Build history of the part. All positions in model axes, mm. A direction names the side the tool comes from. Coordinates: 2 decimals unless noted, no trailing zeros. Loops run counter-clockwise (first coordinate to the right, second up) from the corner with the lowest first, then second, coordinate; pieces in that order, holes last.
(1) Two-plate mould, pull along Y, no slides. Class faces 4 (the face through (45.66, 34.61, 4.93)), 5 (the face through (-0.243, -30.316, 4.93)), 6 (the face through (46.185, -35.23, 4.93)), 7 (the face through (0, 0, 100)): pulls with the +Y half, pulls with the -Y half, needs draft (parallel to the pull), parting line crosses it, or undercut.
(2) Slice it at A-A (x = 0). Give the cut face in (y, z).
(3) Tool access for faces 1 (the face through (-30.57, -55.48, 4.93)), 2 (the face through (-45.66, -34.61, 4.93)), 3 (the face through (6.691, -12.864, 54.37)): list every direction of +Z, -Z, +X, -X, +Y, -Y with a clear straight run to the whole face (end or side of a thin tool).
(4) Slice it at D-D (z = 80). Give the cut face in (x, y).
(5) Slice it at C-C (y = -32.5). Give the cut face in (x, z), and give its area (3 significant figures).
(6) Slice it at B-B (y = 0). Give the cut face in (x, z).
(7) Wall check: L1, parallel to Z at x = 0, y = -1.5; L2, parallel to X at y = -0.5, z = 90.5; L3, parallel to Z at x = -47.5, y = 67. Give the ranges that are in metal, low to high.
(8) Flat gauge pins, fed straight in: P1, Ø6, axis at x = 6.5, z = 75.5, coming from the -Y side; P2, Ø8, axis at x = 25.5, y = 60, coming from the +Z side; P3, Ø16, axis at x = 0, z = 80, coming from the -Y side; P4, Ø6, axis at x = -48, y = 45, coming from the +Z side. Where does each tip first touch, or does it go through?
from build123d import *

# Parameters (mm, degrees)
F1_DEPTH = 10
F3_R     = 14.5
F4_DEPTH = 90
F2_R     = 5
F5_DEPTH = 25


# Not quite as in the source:
# - a feature names something its author has since deleted; it is built from what else it names


with BuildPart() as f1:
    # F0 (on Top) → F1 (new body)
    with BuildSketch(Plane.XY):
        with BuildLine():
            Line((-45.4576714329, 73.0742780183), (-55, 65))
            Line((-55, 65), (-46.9257219817, 55.4576714329))
            ThreePointArc((-46.9257219817, 55.4576714329), (-43.6602805319, 59.7406500035), (-42.5, 65))
            ThreePointArc((-42.5, 65), (-43.2626854202, 69.2994704855), (-45.4576714329, 73.0742780183))
        make_face()
        with BuildLine():
            Line((-46.9257219817, 55.4576714329), (-55, 65))
            Line((-55, 65), (-64.5423285671, 56.9257219817))
            ThreePointArc((-64.5423285671, 56.9257219817), (-56.0380684982, 52.5431780219), (-46.9257219817, 55.4576714329))
        make_face()
        with BuildLine():
            Line((-64.5423285671, 56.9257219817), (-55, 65))
            Line((-55, 65), (-45.4576714329, 73.0742780183))
            ThreePointArc((-45.4576714329, 73.0742780183), (-63.0742780183, 74.5423285671), (-64.5423285671, 56.9257219817))
        make_face()
        with BuildLine():
            ThreePointArc((-42.5, 65), (-43.6602805319, 59.7406500035), (-46.9257219817, 55.4576714329))
            Line((-46.9257219817, 55.4576714329), (-9.3661625013, 11.0691011379))
            ThreePointArc((-9.3661625013, 11.0691011379), (0, 14.5), (9.3661625013, 11.0691011379))
            Line((9.3661625013, 11.0691011379), (46.9257219817, 55.4576714329))
            ThreePointArc((46.9257219817, 55.4576714329), (42.5431780219, 63.9619315018), (45.4576714329, 73.0742780183))
            Line((45.4576714329, 73.0742780183), (15.2677257074, 37.3952512518))
            ThreePointArc((15.2677257074, 37.3952512518), (0, 30.3140960811), (-15.2677257074, 37.3952512518))
            Line((-15.2677257074, 37.3952512518), (-45.4576714329, 73.0742780183))
            ThreePointArc((-45.4576714329, 73.0742780183), (-43.2626854202, 69.2994704855), (-42.5, 65))
        make_face()
        with BuildLine():
            Line((-9.3661625013, 11.0691011379), (-46.9257219817, 55.4576714329))
            ThreePointArc((-46.9257219817, 55.4576714329), (-56.0380684982, 52.5431780219), (-64.5423285671, 56.9257219817))
            Line((-64.5423285671, 56.9257219817), (-27.3057402074, 12.9188448293))
            ThreePointArc((-27.3057402074, 12.9188448293), (-22.5734659148, 0), (-27.3057402074, -12.9188448293))
            Line((-27.3057402074, -12.9188448293), (-64.5423285671, -56.9257219817))
            ThreePointArc((-64.5423285671, -56.9257219817), (-56.0380684982, -52.5431780219), (-46.9257219817, -55.4576714329))
            Line((-46.9257219817, -55.4576714329), (-9.3661625013, -11.0691011379))
            ThreePointArc((-9.3661625013, -11.0691011379), (-14.5, 0), (-9.3661625013, 11.0691011379))
        make_face()
        with BuildLine():
            ThreePointArc((9.3661625013, 11.0691011379), (0, 14.5), (-9.3661625013, 11.0691011379))
            Line((-9.3661625013, 11.0691011379), (0, 0))
            Line((0, 0), (9.3661625013, 11.0691011379))
        make_face()
        with BuildLine():
            Line((0, 0), (-9.3661625013, 11.0691011379))
            ThreePointArc((-9.3661625013, 11.0691011379), (-14.5, 0), (-9.3661625013, -11.0691011379))
            Line((-9.3661625013, -11.0691011379), (0, 0))
        make_face()
        with BuildLine():
            Line((9.3661625013, 11.0691011379), (0, 0))
            Line((0, 0), (9.3661625013, -11.0691011379))
            ThreePointArc((9.3661625013, -11.0691011379), (13.154074583, -6.1008459959), (14.5, 0))
            ThreePointArc((14.5, 0), (13.154074583, 6.1008459959), (9.3661625013, 11.0691011379))
        make_face()
        with BuildLine():
            Line((9.3661625013, -11.0691011379), (0, 0))
            Line((0, 0), (-9.3661625013, -11.0691011379))
            ThreePointArc((-9.3661625013, -11.0691011379), (0, -14.5), (9.3661625013, -11.0691011379))
        make_face()
        with BuildLine():
            Line((46.9257219817, 55.4576714329), (9.3661625013, 11.0691011379))
            ThreePointArc((9.3661625013, 11.0691011379), (13.154074583, 6.1008459959), (14.5, 0))
            ThreePointArc((14.5, 0), (13.154074583, -6.1008459959), (9.3661625013, -11.0691011379))
            Line((9.3661625013, -11.0691011379), (46.9257219817, -55.4576714329))
            ThreePointArc((46.9257219817, -55.4576714329), (56.0380684982, -52.5431780219), (64.5423285671, -56.9257219817))
            Line((64.5423285671, -56.9257219817), (27.3057402074, -12.9188448293))
            ThreePointArc((27.3057402074, -12.9188448293), (22.5734659148, 0), (27.3057402074, 12.9188448293))
            Line((27.3057402074, 12.9188448293), (64.5423285671, 56.9257219817))
            ThreePointArc((64.5423285671, 56.9257219817), (56.0380684982, 52.5431780219), (46.9257219817, 55.4576714329))
        make_face()
        with BuildLine():
            ThreePointArc((9.3661625013, -11.0691011379), (0, -14.5), (-9.3661625013, -11.0691011379))
            Line((-9.3661625013, -11.0691011379), (-46.9257219817, -55.4576714329))
            ThreePointArc((-46.9257219817, -55.4576714329), (-43.6602805319, -59.7406500035), (-42.5, -65))
            ThreePointArc((-42.5, -65), (-43.2626854202, -69.2994704855), (-45.4576714329, -73.0742780183))
            Line((-45.4576714329, -73.0742780183), (-15.2677257074, -37.3952512518))
            ThreePointArc((-15.2677257074, -37.3952512518), (0, -30.3140960811), (15.2677257074, -37.3952512518))
            Line((15.2677257074, -37.3952512518), (45.4576714329, -73.0742780183))
            ThreePointArc((45.4576714329, -73.0742780183), (42.5431780219, -63.9619315018), (46.9257219817, -55.4576714329))
            Line((46.9257219817, -55.4576714329), (9.3661625013, -11.0691011379))
        make_face()
        with BuildLine():
            ThreePointArc((45.4576714329, 73.0742780183), (42.5431780219, 63.9619315018), (46.9257219817, 55.4576714329))
            Line((46.9257219817, 55.4576714329), (55, 65))
            Line((55, 65), (45.4576714329, 73.0742780183))
        make_face()
        with BuildLine():
            Line((55, 65), (46.9257219817, 55.4576714329))
            ThreePointArc((46.9257219817, 55.4576714329), (56.0380684982, 52.5431780219), (64.5423285671, 56.9257219817))
            Line((64.5423285671, 56.9257219817), (55, 65))
        make_face()
        with BuildLine():
            ThreePointArc((-42.5, -65), (-43.6602805319, -59.7406500035), (-46.9257219817, -55.4576714329))
            Line((-46.9257219817, -55.4576714329), (-55, -65))
            Line((-55, -65), (-45.4576714329, -73.0742780183))
            ThreePointArc((-45.4576714329, -73.0742780183), (-43.2626854202, -69.2994704855), (-42.5, -65))
        make_face()
        with BuildLine():
            Line((-55, -65), (-46.9257219817, -55.4576714329))
            ThreePointArc((-46.9257219817, -55.4576714329), (-56.0380684982, -52.5431780219), (-64.5423285671, -56.9257219817))
            Line((-64.5423285671, -56.9257219817), (-55, -65))
        make_face()
        with BuildLine():
            Line((-55, -65), (-64.5423285671, -56.9257219817))
            ThreePointArc((-64.5423285671, -56.9257219817), (-63.0742780183, -74.5423285671), (-45.4576714329, -73.0742780183))
            Line((-45.4576714329, -73.0742780183), (-55, -65))
        make_face()
        with BuildLine():
            ThreePointArc((67.5, 65), (59.2994704855, 76.7373145798), (45.4576714329, 73.0742780183))
            Line((45.4576714329, 73.0742780183), (55, 65))
            Line((55, 65), (64.5423285671, 56.9257219817))
            ThreePointArc((64.5423285671, 56.9257219817), (66.7373145798, 60.7005295145), (67.5, 65))
        make_face()
        with BuildLine():
            ThreePointArc((64.5423285671, -56.9257219817), (56.0380684982, -52.5431780219), (46.9257219817, -55.4576714329))
            Line((46.9257219817, -55.4576714329), (55, -65))
            Line((55, -65), (64.5423285671, -56.9257219817))
        make_face()
        with BuildLine():
            Line((55, -65), (46.9257219817, -55.4576714329))
            ThreePointArc((46.9257219817, -55.4576714329), (42.5431780219, -63.9619315018), (45.4576714329, -73.0742780183))
            Line((45.4576714329, -73.0742780183), (55, -65))
        make_face()
        with BuildLine():
            Line((64.5423285671, -56.9257219817), (55, -65))
            Line((55, -65), (45.4576714329, -73.0742780183))
            ThreePointArc((45.4576714329, -73.0742780183), (59.2994704855, -76.7373145798), (67.5, -65))
            ThreePointArc((67.5, -65), (66.7373145798, -60.7005295145), (64.5423285671, -56.9257219817))
        make_face()
    extrude(amount=F1_DEPTH)

    # F3 (on face) → F4 (join)
    with BuildSketch(Plane.XY.offset(10)):
        Circle(F3_R)
    extrude(amount=F4_DEPTH)

    # F2 (on Front) → F5 (cut, symmetric)
    with BuildSketch(Plane.XZ):
        with Locations((0, 80)):
            Circle(F2_R)
    extrude(amount=F5_DEPTH, both=True, mode=Mode.SUBTRACT)


solid = f1.part
Response values:
1. face 4: undercut
1. face 5: pulls with the -Y half
1. face 6: undercut
1. face 7: needs draft
2. outline: (-30.31, 0) - (30.31, 0) - (30.31, 10) - (14.5, 10) - (14.5, 75) - (-14.5, 75) - (-14.5, 10) - (-30.31, 10) - close; (-14.5, 85) - (14.5, 85) - (14.5, 100) - (-14.5, 100) - close
3. face 1: +Z, -Z, -Y
3. face 2: +Z, -Z, -X
3. face 3: +Z
4. outline: (-5, -13.61) - (-5, 13.61) arc R14.5 ccw to start; (5, -13.61) arc R14.5 ccw to (5, 13.61) - close
5. outline: (-43.87, 0) - (-9.09, 0) - (-9.09, 10) - (-43.87, 10) - close; (9.09, 0) - (43.87, 0) - (43.87, 10) - (9.09, 10) - close
5. area: 696 mm2
6. outline: (-22.57, 0) - (22.57, 0) - (22.57, 10) - (14.5, 10) - (14.5, 100) - (-14.5, 100) - (-14.5, 10) - (-22.57, 10) - close; hole circle Ø10 at (0, 80)
7. L1: z = 0 to 75, 85 to 100
7. L2: x = -14.49 to 14.49
7. L3: z = 0 to 10
8. P1: stops at y = -14.07
8. P2: passes through
8. P3: stops at y = -14.5
8. P4: stops at z = 10
